Geometry: final body of the model. Coordinates: model frame, mm. Face numbers are marked on the shaded views. A direction names the side the tool comes from. Give positions to 0.01 mm unless a question says otherwise; leave off trailing zeros. Order: outer loops, then holes, each group sorted by start corner. A loop starts at its lowest first (then second) coordinate and runs counter-clockwise, first axis right, second up. Notation, with made-up numbers: (-14, 69) - (-7, 69) arc R27 ccw to (-7, 99) - close; hole circle Ø2 at (55.5, 80.25). An arc over 180 degrees is marked (long way). One line per item, written item: value.
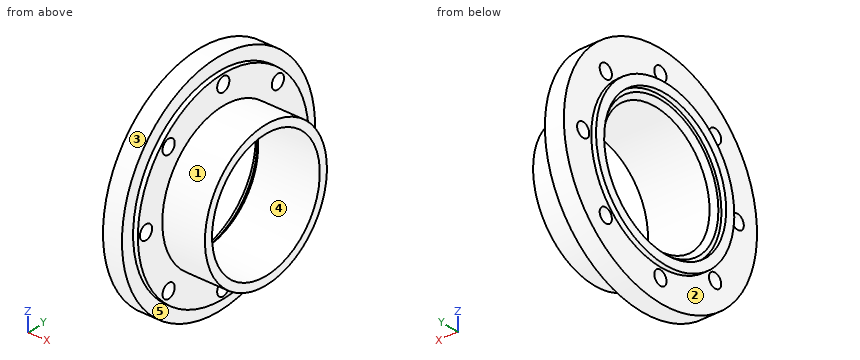
```python
from build123d import *

# Parameters (mm, degrees)
CUT_EXTRUDE_1_REACH = 71.545
SKETCH_3_R          = 3
CHAMFER_1_SIZE      = 2


with BuildPart() as part:
    # 草图1 → 旋转1 (revolve)
    with BuildSketch(Plane.XY, mode=Mode.PRIVATE) as revolve_1_sk:
        Polygon((0, 0), (0, 34), (2, 34), (2, 47.5), (10, 47.5), (10, 42), (12, 42), (12, 30), (30, 30), (30, 0), align=None)
    revolve(revolve_1_sk.sketch.rotate(Axis((0, 0, 0), (-1, 0, 0)), 90), axis=Axis((0, 0, 0), (-1, 0, 0)))

    # 草图2 → 切除-旋转1 (revolve, cut)
    with BuildSketch(Plane.XY, mode=Mode.PRIVATE) as cut_revolve_1_sk:
        Polygon((0, 0), (0, 30), (2, 30), (2, 26.5), (30, 26.5), (30, 0), align=None)
    revolve(cut_revolve_1_sk.sketch.rotate(Axis((0, 0, 0), (-1, 0, 0)), 90), axis=Axis((0, 0, 0), (-1, 0, 0)), mode=Mode.SUBTRACT)

    # 草图3 → 切除-拉伸1 (cut, up to next)
    with BuildSketch(Plane(origin=(12, 0, 0), x_dir=(0, 0, -1), z_dir=(1, 0, 0)), mode=Mode.PRIVATE) as cut_extrude_1_sk1:
        with Locations((0, 38)):
            Circle(SKETCH_3_R)
    cut_extrude_1_tool1 = extrude(cut_extrude_1_sk1.sketch, amount=-CUT_EXTRUDE_1_REACH, mode=Mode.PRIVATE) & part.part
    # 草图3 → 切除-拉伸1 (cut, up to next)
    with BuildSketch(Plane(origin=(12, 0, 0), x_dir=(0, 0, -1), z_dir=(1, 0, 0)), mode=Mode.PRIVATE) as cut_extrude_1_sk2:
        with Locations((26.870057685, 26.870057685)):
            Circle(SKETCH_3_R)
    cut_extrude_1_tool2 = extrude(cut_extrude_1_sk2.sketch, amount=-CUT_EXTRUDE_1_REACH, mode=Mode.PRIVATE) & part.part
    # 草图3 → 切除-拉伸1 (cut, up to next)
    with BuildSketch(Plane(origin=(12, 0, 0), x_dir=(0, 0, -1), z_dir=(1, 0, 0)), mode=Mode.PRIVATE) as cut_extrude_1_sk3:
        with Locations((38, 0)):
            Circle(SKETCH_3_R)
    cut_extrude_1_tool3 = extrude(cut_extrude_1_sk3.sketch, amount=-CUT_EXTRUDE_1_REACH, mode=Mode.PRIVATE) & part.part
    # 草图3 → 切除-拉伸1 (cut, up to next)
    with BuildSketch(Plane(origin=(12, 0, 0), x_dir=(0, 0, -1), z_dir=(1, 0, 0)), mode=Mode.PRIVATE) as cut_extrude_1_sk4:
        with Locations((26.870057685, -26.870057685)):
            Circle(SKETCH_3_R)
    cut_extrude_1_tool4 = extrude(cut_extrude_1_sk4.sketch, amount=-CUT_EXTRUDE_1_REACH, mode=Mode.PRIVATE) & part.part
    # 草图3 → 切除-拉伸1 (cut, up to next)
    with BuildSketch(Plane(origin=(12, 0, 0), x_dir=(0, 0, -1), z_dir=(1, 0, 0)), mode=Mode.PRIVATE) as cut_extrude_1_sk5:
        with Locations((0, -38)):
            Circle(SKETCH_3_R)
    cut_extrude_1_tool5 = extrude(cut_extrude_1_sk5.sketch, amount=-CUT_EXTRUDE_1_REACH, mode=Mode.PRIVATE) & part.part
    # 草图3 → 切除-拉伸1 (cut, up to next)
    with BuildSketch(Plane(origin=(12, 0, 0), x_dir=(0, 0, -1), z_dir=(1, 0, 0)), mode=Mode.PRIVATE) as cut_extrude_1_sk6:
        with Locations((-26.870057685, -26.870057685)):
            Circle(SKETCH_3_R)
    cut_extrude_1_tool6 = extrude(cut_extrude_1_sk6.sketch, amount=-CUT_EXTRUDE_1_REACH, mode=Mode.PRIVATE) & part.part
    # 草图3 → 切除-拉伸1 (cut, up to next)
    with BuildSketch(Plane(origin=(12, 0, 0), x_dir=(0, 0, -1), z_dir=(1, 0, 0)), mode=Mode.PRIVATE) as cut_extrude_1_sk7:
        with Locations((-38, 0)):
            Circle(SKETCH_3_R)
    cut_extrude_1_tool7 = extrude(cut_extrude_1_sk7.sketch, amount=-CUT_EXTRUDE_1_REACH, mode=Mode.PRIVATE) & part.part
    # 草图3 → 切除-拉伸1 (cut, up to next)
    with BuildSketch(Plane(origin=(12, 0, 0), x_dir=(0, 0, -1), z_dir=(1, 0, 0)), mode=Mode.PRIVATE) as cut_extrude_1_sk8:
        with Locations((-26.870057685, 26.870057685)):
            Circle(SKETCH_3_R)
    cut_extrude_1_tool8 = extrude(cut_extrude_1_sk8.sketch, amount=-CUT_EXTRUDE_1_REACH, mode=Mode.PRIVATE) & part.part
    add(cut_extrude_1_tool1.solids().sort_by_distance((12, 38, 0))[0], mode=Mode.SUBTRACT)
    add(cut_extrude_1_tool2.solids().sort_by_distance((12, 26.870058, -26.870058))[0], mode=Mode.SUBTRACT)
    add(cut_extrude_1_tool3.solids().sort_by_distance((12, 0, -38))[0], mode=Mode.SUBTRACT)
    add(cut_extrude_1_tool4.solids().sort_by_distance((12, -26.870058, -26.870058))[0], mode=Mode.SUBTRACT)
    add(cut_extrude_1_tool5.solids().sort_by_distance((12, -38, 0))[0], mode=Mode.SUBTRACT)
    add(cut_extrude_1_tool6.solids().sort_by_distance((12, -26.870058, 26.870058))[0], mode=Mode.SUBTRACT)
    add(cut_extrude_1_tool7.solids().sort_by_distance((12, 0, 38))[0], mode=Mode.SUBTRACT)
    add(cut_extrude_1_tool8.solids().sort_by_distance((12, 26.870058, 26.870058))[0], mode=Mode.SUBTRACT)

    # 倒角1
    chamfer_1_edges = [part.edges().sort_by_distance(p)[0] for p in [
        (2, 0, 26.5),
    ]]
    chamfer(chamfer_1_edges, length=CHAMFER_1_SIZE)


solid = part.part
```
1) Material intervals for line 1 along Y through (x, z) = (17.25, -1); line 2 along Y through (x, z) = (0.8, 0); line 3 along X through (y, z) = (-30, 23.5), sorted ascending.
Answers below:
line 1: -29.98 to -26.48, 26.48 to 29.98
line 2: -34 to -30, 30 to 34
line 3: 2 to 12
2) Mould query, pull axis Y, two halves, no side actions, for the marked faces 3, 4 and 5. Classes: released by +Y, released by -Y, zero draft, split by the parting line, or undercut.
Answers below:
face 3: split by the parting line
face 4: undercut
face 5: zero draft
3) Set-up query: the marked faces 1 and 2. Return all of +Z, -Z, +X, -X, +Y, -Y with unobstructed straight access to the full face (end or side cutting, diameter ignored); none if empty.
Answers below:
face 1: +X
face 2: -X
4) First-contact query: pin 1 (12 mm diameter, centred on y = 26, z = 38, fed in from +X); pin 2 (5 mm diameter, centred on x = 13.5, y = -21.5, fed in from -Z); pin 3 (4 mm diameter, centred on x = 8.5, z = 6, fed in from +Y). Flat tips, straight axial feed; report the tip coordinate or a pass-through.
Answers below:
pin 1: x = 12
pin 2: z = -37.2
pin 3: y = 47.33
5) Section B-B, the plane y = 0. Count the separate pieces of the cut face and the enclosed holes in it, then the cut area to 3 significant figures.
Answers below:
separate pieces: 4
enclosed holes: 0
area: 416 mm^2
6) Section A-A, the plane y = 38. Return loops of the section in (x, z), then the cut area to 3 significant figures.
Answers below:
outline: (2, -28.5) - (10, -28.5) - (10, -17.89) - (12, -17.89) - (12, -3) - (2, -3) - close; (2, 3) - (12, 3) - (12, 17.89) - (10, 17.89) - (10, 28.5) - (2, 28.5) - close
area: 468 mm^2
7) Section D-D, the plane x = 17.25. Return loops of the section in (y, z).
Answers below:
outline: circle Ø60 at (0, 0); hole circle Ø53 at (0, 0)
